The listing builds one solid part. Answer for the finished solid, in the listing's coordinates (mm). A direction names the side the tool comes from. Give positions to 0.01 mm unless a question says otherwise; leave off trailing zeros. Order: outer loops, then holes, each group sorted by start corner. A loop starts at its lowest first (then second) coordinate and runs counter-clockwise, first axis right, second up. Notation, with made-up numbers: (59.25, 25.25) - (63.25, 25.25) arc R32 cw to (63.25, 56.25) - close; hole circle Ø6 at (36, 51.25). An arc over 180 degrees is marked (long way). Answer as a JSON object with one key per item and string values. Group by question number.
Q1. A cutting plane is placed at A-A, the plane z = -3. Give the vertices of the cut face in (x, y), and give its area (3 significant figures).
Q2. A cutting plane is placed at B-B, the plane z = -19.5. Give the vertices of the cut face in (x, y), and give its area (3 significant figures).
Q3. Consider line 1 (Y direction, x = 72.5, z = -33); line 2 (Y direction, x = -90, z = -1.5); line 3 (Z direction, x = 7, y = -7). Determine where each line is inside the solid, lowest interval first.
Q4. For faces 5 (the face through (78, -3.329, -26)), 6 (the face through (1, -40.688, 1)), 7 (the face through (1, -43.688, -7)), determine the directions among +Z, -Z, +X, -X, +Y, -Y from which every point of the face is accessible in a straight line to the end or side of a thin tool.
Q5. The mould has two halves that part along X. Classify faces 1 (the face through (-55.653, -22, -13)), 2 (the face through (1, -3, 1)), 3 (the face through (55.653, -22, -13)), 4 (the face through (-100, -22, -11)): released by +X, released by -X, zero draft, split by the parting line, or undercut.
Q6. Given pin 1 (1 mm diameter, centred on x = -5, y = -9.5, fed in from -Z); pin 2 (6 mm diameter, centred on x = -30, y = -36.5, fed in from +Z); pin 3 (11 mm diameter, centred on x = -77.5, y = -20, fed in from -Z), each flat-ended and moving along its own axis, determine where each tip first touches the part or whether it passes through.
Q7. A cutting plane is placed at D-D, the plane y = -10.5. Give the vertices of the cut face in (x, z), and give its area (4 significant figures).
Q8. A cutting plane is placed at C-C, the plane x = -71.5. Give the vertices of the cut face in (y, z).
from build123d import *

# Parameters (mm, degrees)
F0_W     = 200
F0_H     = 25
F1_DEPTH = 43.688
F2_W     = 37.688
F2_H     = 22
F3_DEPTH = 200.001
F4_W     = 44.3474374712
F4_H     = 43.688
F5_DEPTH = 25
F7_W     = 36.9936539792
F7_H     = 24.3178982288
F8_DEPTH = 200.001


with BuildPart() as f1:
    # F0 (on Front) → F1 (new body)
    with BuildSketch(Plane.XZ):
        Rectangle(F0_W, F0_H)
    extrude(amount=F1_DEPTH)

    # F2 (on face) → F3 (cut, through all)
    with BuildSketch(Plane.YZ.offset(100)):
        with Locations((-21.844, 1.5)):
            Rectangle(F2_W, F2_H)
    extrude(amount=-F3_DEPTH, mode=Mode.SUBTRACT)

    # F4 (on face) → F5 (join)
    with BuildSketch(Plane(origin=(0, 0, -12.5), x_dir=(1, 0, 0), z_dir=(0, 0, -1))):
        with Locations((77.8262812644, 21.844)):
            Rectangle(F4_W, F4_H)
    extrude(amount=F5_DEPTH)

    # F6: F1 across plane


with BuildPart() as f1_1:
    add(f1.part)
    add(f1.part.mirror(Plane.YZ))

    # F7 (on face) → F8 (cut, through all)
    with BuildSketch(Plane.YZ.offset(100)):
        with Locations((-21.8255401123, -25.3410508856)):
            Rectangle(F7_W, F7_H)
    extrude(amount=-F8_DEPTH, mode=Mode.SUBTRACT)


solid = f1_1.part
Reply:
{
 "1": {"outline": "(-100, -43.69) - (100, -43.69) - (100, -40.69) - (-100, -40.69) - close; (-100, -3) - (100, -3) - (100, 0) - (-100, 0) - close", "area": "1,200 mm^2"},
 "2": {"outline": "(-100, -43.69) - (-55.65, -43.69) - (-55.65, -40.32) - (-100, -40.32) - close; (-100, -3.33) - (-55.65, -3.33) - (-55.65, 0) - (-100, 0) - close; (55.65, -43.69) - (100, -43.69) - (100, -40.32) - (55.65, -40.32) - close; (55.65, -3.33) - (100, -3.33) - (100, 0) - (55.65, 0) - close", "area": "594 mm^2"},
 "3": {"line 1": "y = -43.69 to -40.32, -3.33 to 0", "line 2": "y = -43.69 to -40.69, -3 to 0", "line 3": "z = -12.5 to -9.5"},
 "4": {"face 5": "-Z, +X, -X", "face 6": "+Z, +X, -X", "face 7": "+Z, -Z, +X, -X, -Y"},
 "5": {"face 1": "undercut", "face 2": "zero draft", "face 3": "undercut", "face 4": "released by -X"},
 "6": {"pin 1": "stops at z = -12.5", "pin 2": "stops at z = -9.5", "pin 3": "stops at z = -13.18"},
 "7": {"outline": "(-100, -13.18) - (-55.65, -13.18) - (-55.65, -12.5) - (55.65, -12.5) - (55.65, -13.18) - (100, -13.18) - (100, -9.5) - (-100, -9.5) - close", "area": "660.5 mm^2"},
 "8": {"outline": "(-43.69, -37.5) - (-40.32, -37.5) - (-40.32, -13.18) - (-3.33, -13.18) - (-3.33, -37.5) - (0, -37.5) - (0, 12.5) - (-3, 12.5) - (-3, -9.5) - (-40.69, -9.5) - (-40.69, 12.5) - (-43.69, 12.5) - close"}
}
